Geometry check sheet. Reference: the model listing, model coordinates, mm. Coordinates: 2 decimals unless noted, no trailing zeros. Write each loop counter-clockwise with the first axis right and the second up, starting at its lowest first coordinate (ties: lowest second). Pieces come first, ordered by that corner, then holes.
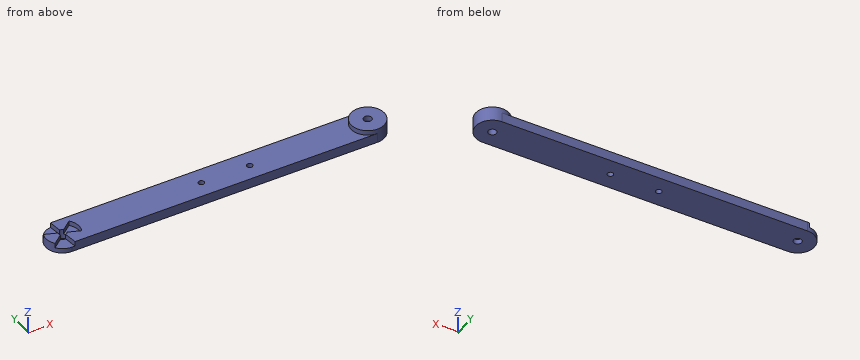
from build123d import *
from build123d.topology import SkipClean

# Parameters (mm, degrees)
SKETCH1_R            = 2.5
BOSS_EXTRUDE1_DEPTH  = 6
CUT_EXTRUDE3_DEPTH   = 3
BOSS_EXTRUDE2_START  = 3
SKETCH4_R            = 2.5
BOSS_EXTRUDE2_DEPTH  = 3
M3_CLEARANCE_HOLE1_D = 3.6


with BuildPart() as part:
    # Sketch1 → Boss-Extrude1 (new body)
    with BuildSketch(Plane.XY):
        with BuildLine():
            Line((189.7, -10.4), (0, -10.4))
            ThreePointArc((0, -10.4), (-10.4, 0), (0, 10.4))
            Line((0, 10.4), (189.7, 10.4))
            ThreePointArc((189.7, 10.4), (200.1, 0), (189.7, -10.4))
        make_face()
        Circle(SKETCH1_R, mode=Mode.SUBTRACT)
        with Locations((189.7, 0)):
            Circle(SKETCH1_R, mode=Mode.SUBTRACT)
    extrude(amount=BOSS_EXTRUDE1_DEPTH)

    # Sketch6 → Cut-Extrude3 (cut)
    with BuildSketch(Plane(origin=(0, 0, 0), x_dir=(-1, 0, 0), z_dir=(0, 0, -1))):
        with BuildLine():
            ThreePointArc((0.189684667, 2.492793559), (1.571265552, 1.944511395), (2.39740304, 0.708843186))
            Line((2.39740304, 0.708843186), (9.962077265, 3.621742201))
            ThreePointArc((9.962077265, 3.621742201), (6.66216594, 8.244728315), (1.449377234, 10.500443116))
            Line((1.449377234, 10.500443116), (0.189684667, 2.492793559))
        make_face()
        with BuildLine():
            ThreePointArc((2.063980215, -1.41066852), (0.89836349, -2.333011582), (-0.584825314, -2.430633529))
            Line((-0.584825314, -2.430633529), (-1.844517881, -10.438283086))
            ThreePointArc((-1.844517881, -10.438283086), (3.809061198, -9.891969106), (8.368961872, -6.505419062))
            Line((8.368961872, -6.505419062), (2.063980215, -1.41066852))
        make_face()
        with BuildLine():
            Line((-9.818339107, -3.995024054), (-2.253664882, -1.082125039))
            ThreePointArc((-2.253664882, -1.082125039), (-2.469629042, 0.388500187), (-1.812577726, 1.721790343))
            Line((-1.812577726, 1.721790343), (-8.117559384, 6.816540886))
            ThreePointArc((-8.117559384, 6.816540886), (-10.471227138, 1.647240791), (-9.818339107, -3.995024054))
        make_face()
    extrude(amount=-CUT_EXTRUDE3_DEPTH, mode=Mode.SUBTRACT)

    # Sketch4 → Boss-Extrude2 (add)
    with SkipClean():  # the faces are left unmerged after this step: merging them gives an invalid solid
        with BuildSketch(Plane(origin=(0, 0, 0), x_dir=(-1, 0, 0), z_dir=(0, 0, -1)).offset(BOSS_EXTRUDE2_START)):
            with BuildLine():
                ThreePointArc((-189.7, 10.4), (-200.1, 0), (-189.7, -10.4))
                ThreePointArc((-189.7, -10.4), (-179.3, 0), (-189.7, 10.4))
            make_face()
            with Locations((-189.7, 0)):
                Circle(SKETCH4_R, mode=Mode.SUBTRACT)
        extrude(amount=-BOSS_EXTRUDE2_DEPTH)


with BuildPart() as body_2:
    # Mirror1: mirrored copy
    add(part.part.mirror(Plane.XY))

    # M3 Clearance Hole1 (through all)
    with Locations(Plane(origin=(0, 0, -6), x_dir=(-1, 0, 0), z_dir=(0, 0, -1))):
        with Locations((-116.336074354, -0.050784287), (-86.336165629, 0.001543951)):
            Hole(M3_CLEARANCE_HOLE1_D / 2)


solid = body_2.part
1. Sectioned sample at B-B, the plane x = 137. Record the boundary of the cut face in (y, z), and give its area (3 significant figures).
Computed values:
outline: (-10.4, -6) - (10.4, -6) - (10.4, 0) - (-10.4, 0) - close
area: 125 mm2
2. Gauge pin test, flat ends, axial feed: pin 1 Ø3 at (y, z) = (8, 1.5) entering from +X; pin 2 Ø2.5 at (x, y) = (5, 2) entering from +Z; pin 3 Ø5 at (x, y) = (163, 2) entering from +Z. Record the tip position at first contact, or that the pin passes through.
Computed values:
pin 1: stops at x = 197.82
pin 2: stops at z = -3
pin 3: stops at z = 0
3. Sectioned sample at A-A, the plane x = 4.5. Record the boundary of the cut face in (y, z).
Computed values:
outline: (-10.4, -6) - (10.4, -6) - (10.4, 0) - (3.89, 0) - (3.89, -3) - (-1.95, -3) - (-1.95, 0) - (-10.4, 0) - close
4. Thickness scan on line 1 along X through (y, z) = (0, -2.3); line 2 along Z through (x, y) = (153.5, 8.25); line 3 along X through (y, z) = (0, 1.1). Record the ranges inside material, lowest first.
Computed values:
line 1: x = -10.4 to -2.5, 10.6 to 84.54, 88.14 to 114.54, 118.14 to 187.2, 192.2 to 200.1
line 2: z = -6 to 0
line 3: x = 179.3 to 187.2, 192.2 to 200.1
